from build123d import *

# Parameters (mm, degrees)
SKETCH1_W           = 76.2
SKETCH1_H           = 15.24
BOSS_EXTRUDE1_DEPTH = 5.08
SKETCH2_W           = 25.4
SKETCH2_H           = 5.08
BOSS_EXTRUDE2_DEPTH = 31.75
SKETCH4_W           = 5.08
SKETCH4_H           = 19.05
CUT_EXTRUDE2_DEPTH  = 50.8
SKETCH6_W           = 5.08
SKETCH6_H           = 34.29
BOSS_EXTRUDE3_DEPTH = 19.05
SKETCH7_W           = 5.08
SKETCH7_H           = 19.05
CUT_EXTRUDE4_DEPTH  = 19.05
FILLET1_R           = 12.7
SKETCH12_W          = 5.08
SKETCH12_H          = 5.08
BOSS_EXTRUDE5_DEPTH = 3.81
SKETCH14_W          = 31.440322014
SKETCH14_H          = 5.08
BOSS_EXTRUDE7_DEPTH = 1.27
CUT_EXTRUDE7_DEPTH  = 50.854577523
FILLET3_R           = 17.78


with BuildPart() as part:
    # Sketch1 → Boss-Extrude1 (new body)
    with BuildSketch(Plane.XY):
        Rectangle(SKETCH1_W, SKETCH1_H)
    extrude(amount=BOSS_EXTRUDE1_DEPTH)

    # Sketch2 → Boss-Extrude2 (add)
    with BuildSketch(Plane(origin=(0, 0, 0), x_dir=(1, 0, 0), z_dir=(0, 1, 0))):
        with Locations((-6.35, -2.54)):
            Rectangle(SKETCH2_W, SKETCH2_H)
    extrude(amount=BOSS_EXTRUDE2_DEPTH)

    # Sketch4 → Cut-Extrude2 (cut)
    with BuildSketch(Plane(origin=(0, 0, 0), x_dir=(-1, 0, 0), z_dir=(0, 0, -1))):
        with Locations((6.35, 14.605)):
            Rectangle(SKETCH4_W, SKETCH4_H)
    extrude(amount=-CUT_EXTRUDE2_DEPTH, mode=Mode.SUBTRACT)

    # Sketch6 → Boss-Extrude3 (add)
    with BuildSketch(Plane.ZY.offset(19.05)):
        with Locations((2.54, 14.605)):
            Rectangle(SKETCH6_W, SKETCH6_H)
    extrude(amount=BOSS_EXTRUDE3_DEPTH)

    # Sketch7 → Cut-Extrude4 (cut)
    with BuildSketch(Plane(origin=(0, 0, 0), x_dir=(-1, 0, 0), z_dir=(0, 0, -1))):
        with Locations((16.51, 14.605)):
            Rectangle(SKETCH7_W, SKETCH7_H)
    extrude(amount=-CUT_EXTRUDE4_DEPTH, mode=Mode.SUBTRACT)

    # Fillet1
    fillet1_edges = [part.edges().sort_by_distance(p)[0] for p in [
        (6.35, 31.75, 2.54),
        (-38.1, 31.75, 2.54),
    ]]
    fillet(fillet1_edges, radius=FILLET1_R)

    # Sketch12 → Boss-Extrude5 (add)
    with BuildSketch(Plane.XZ.offset(7.62)):
        with Locations((35.56, 2.54)):
            Rectangle(SKETCH12_W, SKETCH12_H)
    extrude(amount=BOSS_EXTRUDE5_DEPTH)

    # Sketch14 → Boss-Extrude7 (add)
    with BuildSketch(Plane.XZ.offset(7.62)):
        with Locations((17.299838993, 2.54)):
            Rectangle(SKETCH14_W, SKETCH14_H)
    extrude(amount=BOSS_EXTRUDE7_DEPTH)

    # Sketch9 → Cut-Extrude7 (cut, through all)
    with BuildSketch(Plane.XY.offset(5.08)):
        with BuildLine():
            Line((22.048333309, -23.322415838), (-34.748333309, -23.322415838))
            ThreePointArc((-34.748333309, -23.322415838), (-25.400905918, -5.197262826), (-6.35, 2.08))
            ThreePointArc((-6.35, 2.08), (12.700905918, -5.197262826), (22.048333309, -23.322415838))
        make_face()
    extrude(amount=-CUT_EXTRUDE7_DEPTH, mode=Mode.SUBTRACT)

    # Fillet3
    fillet3_edges = [part.edges().sort_by_distance(p)[0] for p in [
        (38.1, 7.62, 2.54),
    ]]
    fillet(fillet3_edges, radius=FILLET3_R)


solid = part.part
Input: part model. Units: mm. Frame: model coordinates. A direction names the side the tool comes from. Round coordinates to 2 decimals unless told otherwise and drop trailing zeros. Loops run counter-clockwise (first coordinate to the right, second up) from the corner with the lowest first, then second, coordinate; pieces in that order, holes last. Notation, with made-up numbers: M -30,-22 L 16,-22 A28 cw 16,5 Z; hole C 16.25,33.25 d7. An arc over 180 degrees is marked long. Answer as CSV lines item,"result". Start each with the question number.
(1) Section A-A, the plane y = 18. Output: boundary loops of the cut face in (x, z), plus the area to 3 significant figures.
(2) Section C-C, the plane x = -7.5. Output: boundary loops of the cut face in (y, z), plus the area to 3 significant figures.
(3) Section B-B, the plane z = 2.45. Output: boundary loops of the cut face in (x, y) (3 decimals), plus the area to 3 significant figures.
(4) Section D-D, the plane y = -5. Output: boundary loops of the cut face in (x, z).
(5) Reachability of faces 4 (the flat face through (33.02, -10, 3)), 5 (the flat face through (13, 7.62, 3)), 6 (the flat face through (-13.97, 14, 3)) from +Z, -Z, +X, -X, +Y, -Y: full face, straight path, thin tool, end or side. Return the list, or none.
(6) Draft query along Y for faces 1 (the cylindrical face through (-34.48, 27.93, 2.58)), 2 (the flat face through (-3.81, 14, 3)), 3 (the flat face through (-33, -7.62, 3)). Return one class per face: released by +Y, released by -Y, zero draft, split by the parting line, or undercut.
(7) Line query: line 1 (X direction, y = 18.5, z = 4.65); line 2 (X direction, y = 21, z = 0.8); line 3 (X direction, y = 28, z = 1.35). Output: solid intervals per line, ascending. Write a range as [from, to].
(8) First-contact query: pin 1 (3 mm diameter, centred on x = 20, z = 3.5, fed in from -Y); pin 2 (2.5 mm diameter, centred on x = -7.5, z = 1.5, fed in from -Y); pin 3 (1.5 mm diameter, centred on x = -32, z = 1.5, fed in from -Y). Flat tips, straight axial feed; report the tip coordinate or a pass-through.
Values found:
1,outline,"M -38.1,0 L -19.05,0 L -19.05,5.08 L -38.1,5.08 Z; M -13.97,0 L -8.89,0 L -8.89,5.08 L -13.97,5.08 Z; M -3.81,0 L 6.35,0 L 6.35,5.08 L -3.81,5.08 Z"
1,area,"174 mm²"
2,outline,"M 2.06,0 L 5.08,0 L 5.08,5.08 L 2.06,5.08 Z; M 24.13,0 L 31.75,0 L 31.75,5.08 L 24.13,5.08 Z"
2,area,"54.1 mm²"
3,outline,"M -38.1,-7.62 L -27.804,-7.62 A28.575 cw 16.158,-8.89 L 33.02,-8.89 L 33.02,-11.43 L 38.1,-11.43 L 38.1,-10.16 A17.78 ccw 20.32,7.62 L 6.35,7.62 L 6.35,19.05 A12.7 ccw -6.35,31.75 L -25.4,31.75 A12.7 ccw -38.1,19.05 Z; hole M -19.05,5.08 L -13.97,5.08 L -13.97,24.13 L -19.05,24.13 Z; hole M -8.89,5.08 L -3.81,5.08 L -3.81,24.13 L -8.89,24.13 Z"
3,area,"1,660 mm²"
4,outline,"M -38.1,0 L -25.18,0 L -25.18,5.08 L -38.1,5.08 Z; M 12.48,0 L 37.33,0 L 37.33,5.08 L 12.48,5.08 Z"
5,face 4,"+Z, -Z, -X, -Y"
5,face 5,"+Z, -Z, +X, +Y"
5,face 6,"+Z, -Z"
6,face 1,"released by +Y"
6,face 2,"undercut"
6,face 3,"released by -Y"
7,line 1,"x = [-38.1, -19.05], [-13.97, -8.89], [-3.81, 6.35]"
7,line 2,"x = [-37.95, -19.05], [-13.97, -8.89], [-3.81, 6.2]"
7,line 3,"x = [-34.41, 2.66]"
8,pin 1,"stops at y = -8.89"
8,pin 2,"stops at y = 1.98"
8,pin 3,"stops at y = -7.62"
